from build123d import *

# Parameters (mm, degrees)
SKETCH_1_R          = 42.5
SKETCH_1_R_2        = 3
EXTRUDE_1_DEPTH     = 6
SKETCH_1_3_R        = 42.5
SKETCH_1_3_R_2      = 37.5
EXTRUDE_2_DEPTH     = 62
EXTRUDE_START       = 37
SKETCH_1_5_R        = 37.5
SKETCH_1_5_R_2      = 20
EXTRUDE_3_DEPTH     = 5
CHAMFER_1_SIZE      = 2
EXTRUDE_4_DEPTH     = 37
CUT_EXTRUDE_2_DEPTH = 25
CUT_EXTRUDE_3_REACH = 78.25


with BuildPart() as part:
    # 草图1 → 凸台-拉伸1 (new body)
    with BuildSketch(Plane(origin=(0, 0, 0), x_dir=(1, 0, 0), z_dir=(0, 1, 0))):
        with BuildLine():
            Line((-36, 45), (36, 45))
            ThreePointArc((36, 45), (42.363961031, 42.363961031), (45, 36))
            Line((45, 36), (45, -36))
            ThreePointArc((45, -36), (42.363961031, -42.363961031), (36, -45))
            Line((36, -45), (-36, -45))
            ThreePointArc((-36, -45), (-42.363961031, -42.363961031), (-45, -36))
            Line((-45, -36), (-45, 36))
            ThreePointArc((-45, 36), (-42.363961031, 42.363961031), (-36, 45))
        make_face()
        with Locations(Location((0, 0, 0), (0, 0, 270))):
            Circle(SKETCH_1_R, mode=Mode.SUBTRACT)
        with Locations(Location((-36, 36, 0), (0, 0, 270))):
            Circle(SKETCH_1_R_2, mode=Mode.SUBTRACT)
        with Locations(Location((36, 36, 0), (0, 0, 270))):
            Circle(SKETCH_1_R_2, mode=Mode.SUBTRACT)
        with Locations(Location((36, -36, 0), (0, 0, 270))):
            Circle(SKETCH_1_R_2, mode=Mode.SUBTRACT)
        with Locations(Location((-36, -36, 0), (0, 0, 270))):
            Circle(SKETCH_1_R_2, mode=Mode.SUBTRACT)
    extrude(amount=EXTRUDE_1_DEPTH)

    # 草图1<3> → 凸台-拉伸2 (add)
    with BuildSketch(Plane(origin=(0, 0, 0), x_dir=(1, 0, 0), z_dir=(0, 1, 0))):
        with Locations(Location((0, 0, 0), (0, 0, 270))):
            Circle(SKETCH_1_3_R)
        with Locations(Location((0, 0, 0), (0, 0, 270))):
            Circle(SKETCH_1_3_R_2, mode=Mode.SUBTRACT)
    extrude(amount=EXTRUDE_2_DEPTH)

    # 草图1<5> → 凸台-拉伸3 (add)
    with BuildSketch(Plane(origin=(0, 0, 0), x_dir=(1, 0, 0), z_dir=(0, 1, 0)).offset(EXTRUDE_START)):
        with Locations(Location((0, 0, 0), (0, 0, 270))):
            Circle(SKETCH_1_5_R)
        with Locations(Location((0, 0, 0), (0, 0, 270))):
            Circle(SKETCH_1_5_R_2, mode=Mode.SUBTRACT)
    extrude(amount=EXTRUDE_3_DEPTH)

    # 倒角1
    chamfer_1_edges = [part.edges().sort_by_distance(p)[0] for p in [
        (0, 42, -20),
    ]]
    chamfer(chamfer_1_edges, length=CHAMFER_1_SIZE)

    # 草图1<6> → 凸台-拉伸4 (add)
    with BuildSketch(Plane(origin=(0, 0, 0), x_dir=(1, 0, 0), z_dir=(0, 1, 0))):
        with BuildLine():
            Line((27.950849719, -25), (-27.950849719, -25))
            ThreePointArc((-27.950849719, -25), (0, -37.5), (27.950849719, -25))
        make_face()
    extrude(amount=EXTRUDE_4_DEPTH)

    # 草图2 → 切除-拉伸2 (cut)
    with BuildSketch(Plane(origin=(0, 6, 0), x_dir=(1, 0, 0), z_dir=(0, 1, 0))):
        with BuildLine():
            Line((-27.882352941, -27.978999168), (-30, -30.103986447))
            ThreePointArc((-30, -30.103986447), (0, -42.5), (30, -30.103986447))
            Line((30, -30.103986447), (27.882352941, -27.978999168))
            ThreePointArc((27.882352941, -27.978999168), (0, -39.5), (-27.882352941, -27.978999168))
        make_face()
    extrude(amount=CUT_EXTRUDE_2_DEPTH, mode=Mode.SUBTRACT)

    # 草图3 → 切除-旋转1 (revolve, cut)
    with BuildSketch(Plane(origin=(0, 18.5, 0), x_dir=(1, 0, 0), z_dir=(0, 1, 0))):
        Polygon((11.657691454, -25), (17.095538176, -22.46429043), (18.961631098, -26.466139615), (15.789553843, -27.945303531), (20.195943791, -37.394837269), (17.930174324, -38.451382923), align=None)
    revolve(axis=Axis((17.930174324, 18.5, 38.451382923), (-0.42261826174070033, 0, -0.9063077870366495)), mode=Mode.SUBTRACT)

    # 草图3<4> → 切除-旋转2 (revolve, cut)
    with BuildSketch(Plane(origin=(0, 18.5, 0), x_dir=(1, 0, 0), z_dir=(0, 1, 0)), mode=Mode.PRIVATE) as cut_revolve_2_sk:
        Polygon((-20.195943791, -37.394837269), (-17.930174324, -38.451382923), (-11.657691454, -25), (-17.095538176, -22.46429043), (-18.961631098, -26.466139615), (-15.789553843, -27.945303531), align=None)
    revolve(cut_revolve_2_sk.sketch.rotate(Axis((-17.930174324, 18.5, 38.451382923), (0.42261826174069994, 0, -0.9063077870366497)), 180), axis=Axis((-17.930174324, 18.5, 38.451382923), (0.42261826174069994, 0, -0.9063077870366497)), mode=Mode.SUBTRACT)

    # 草图5 → 切除-拉伸3 (cut, up to next)
    with BuildSketch(Plane(origin=(0, 42, 0), x_dir=(1, 0, 0), z_dir=(0, 1, 0)), mode=Mode.PRIVATE) as cut_extrude_3_sk1:
        with BuildLine():
            Line((-6, 30), (-2.872281323, 30))
            ThreePointArc((-2.872281323, 30), (0, 31.5), (2.872281323, 30))
            Line((2.872281323, 30), (6, 30))
            ThreePointArc((6, 30), (8, 28), (6, 26))
            Line((6, 26), (2.872281323, 26))
            ThreePointArc((2.872281323, 26), (0, 24.5), (-2.872281323, 26))
            Line((-2.872281323, 26), (-6, 26))
            ThreePointArc((-6, 26), (-8, 28), (-6, 30))
        make_face()
    cut_extrude_3_tool1 = extrude(cut_extrude_3_sk1.sketch, amount=-CUT_EXTRUDE_3_REACH, mode=Mode.PRIVATE) & part.part
    # 草图5 → 切除-拉伸3 (cut, up to next)
    with BuildSketch(Plane(origin=(0, 42, 0), x_dir=(1, 0, 0), z_dir=(0, 1, 0)), mode=Mode.PRIVATE) as cut_extrude_3_sk2:
        with BuildLine():
            Line((26, 6), (26, 2.872281323))
            ThreePointArc((26, 2.872281323), (24.5, 0), (26, -2.872281323))
            Line((26, -2.872281323), (26, -6))
            ThreePointArc((26, -6), (28, -8), (30, -6))
            Line((30, -6), (30, -2.872281323))
            ThreePointArc((30, -2.872281323), (31.5, 0), (30, 2.872281323))
            Line((30, 2.872281323), (30, 6))
            ThreePointArc((30, 6), (28, 8), (26, 6))
        make_face()
    cut_extrude_3_tool2 = extrude(cut_extrude_3_sk2.sketch, amount=-CUT_EXTRUDE_3_REACH, mode=Mode.PRIVATE) & part.part
    # 草图5 → 切除-拉伸3 (cut, up to next)
    with BuildSketch(Plane(origin=(0, 42, 0), x_dir=(1, 0, 0), z_dir=(0, 1, 0)), mode=Mode.PRIVATE) as cut_extrude_3_sk3:
        with BuildLine():
            Line((-26, -6), (-26, -2.872281323))
            ThreePointArc((-26, -2.872281323), (-24.5, 0), (-26, 2.872281323))
            Line((-26, 2.872281323), (-26, 6))
            ThreePointArc((-26, 6), (-28, 8), (-30, 6))
            Line((-30, 6), (-30, 2.872281323))
            ThreePointArc((-30, 2.872281323), (-31.5, 0), (-30, -2.872281323))
            Line((-30, -2.872281323), (-30, -6))
            ThreePointArc((-30, -6), (-28, -8), (-26, -6))
        make_face()
    cut_extrude_3_tool3 = extrude(cut_extrude_3_sk3.sketch, amount=-CUT_EXTRUDE_3_REACH, mode=Mode.PRIVATE) & part.part
    add(cut_extrude_3_tool1.solids().sort_by_distance((0, 42, -28))[0], mode=Mode.SUBTRACT)
    add(cut_extrude_3_tool2.solids().sort_by_distance((28, 42, 0))[0], mode=Mode.SUBTRACT)
    add(cut_extrude_3_tool3.solids().sort_by_distance((-28, 42, 0))[0], mode=Mode.SUBTRACT)


solid = part.part
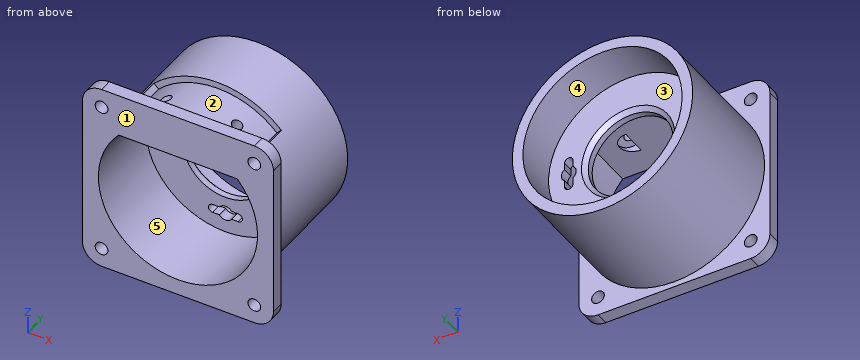
Input: part model. Units: mm. Frame: model coordinates. Face numbers are marked on the shaded views. A direction names the side the tool comes from. Give positions to 0.01 mm unless a question says otherwise; leave off trailing zeros. Order: outer loops, then holes, each group sorted by start corner. A loop starts at its lowest first (then second) coordinate and runs counter-clockwise, first axis right, second up. Notation, with made-up numbers: (85, -16) - (105, -16) arc R29 ccw to (105, 14) - close; hole circle Ø8 at (58, -22). An arc over 180 degrees is marked (long way). Answer as a JSON object with one key per item and string values. Group by question number.
Q1. Cut plane D-D, the plane y = 14. Output: boundary loops of the cut face in (x, z).
Q2. Cut plane A-A, the plane x = 0. Output: boundary loops of the cut face in (y, z).
Q3. Cut plane C-C, the plane y = 32.5. Output: boundary loops of the cut face in (x, z).
Q4. Line query: probe 1 along X at (y, z) = (1, 36); probe 2 along X at (y, z) = (22, 0); probe 3 along Y at (x, z) = (12.5, 40). Output: solid intervals per line, ascending.
Q5. First-contact query: pin 1 Ø3.5 at (y, z) = (39, -4.5) entering from -X; pin 2 Ø0.9 at (x, y) = (3.5, 40.5) entering from -Z; pin 3 Ø0.9 at (y, z) = (40, -5) entering from +X; pin 4 Ø5 at (x, z) = (-36, -36) entering from +Y. Flat tips, straight axial feed; report the tip coordinate or a pass-through.
Q6. Mould query, pull axis Z, two halves, no side actions, for the marked faces 1, 2 and 3. Classes: pulls with the +Z half, pulls with the -Z half, needs draft (parallel to the pull), parting line crosses it, or undercut.
Q7. Set-up query: the marked faces 4 and 5. Return all of +Z, -Z, +X, -X, +Y, -Y with unobstructed straight access to the full face (end or side cutting, diameter ignored); none if empty.
Q8. Cut plane B-B, the plane z = -28. Output: boundary loops of the cut face in (x, y), then the cut area to 3 significant figures.
Results:
{
 "1": {"outline": "(-30, 30.1) arc R42.5 ccw (long way) to (30, 30.1) - (27.88, 27.98) arc R39.5 ccw to (-27.88, 27.98) - close; hole (-27.95, 25) arc R37.5 ccw (long way) to (27.95, 25) - (16.04, 25) - (17.12, 27.32) - (9.93, 30.68) - (8.06, 26.68) - (11.66, 25) - (-11.66, 25) - (-8.06, 26.68) - (-9.93, 30.68) - (-17.12, 27.32) - (-16.04, 25) - close"},
 "2": {"outline": "(0, -45) - (6, -45) - (6, -42.5) - (62, -42.5) - (62, -37.5) - (42, -37.5) - (42, -31.5) - (37, -31.5) - (37, -37.5) - (0, -37.5) - close; (0, 25) - (37, 25) - (37, 20) - (40, 20) - (42, 22) - (42, 37.5) - (62, 37.5) - (62, 42.5) - (31, 42.5) - (31, 39.5) - (6, 39.5) - (6, 45) - (0, 45) - close; (37, -24.5) - (42, -24.5) - (42, -22) - (40, -20) - (37, -20) - close"},
 "3": {"outline": "circle Ø85 at (0, 0); hole (-27.95, 25) arc R37.5 ccw (long way) to (27.95, 25) - close"},
 "4": {"probe 1": "-45 to -39, -33 to 33, 39 to 45", "probe 2": "-42.5 to -37.5, 37.5 to 42.5", "probe 3": "0 to 6, 31 to 62"},
 "5": {"pin 1": "x = -42.41", "pin 2": "z = -42.39", "pin 3": "x = 42.26", "pin 4": "through"},
 "6": {"face 1": "needs draft", "face 2": "pulls with the +Z half", "face 3": "undercut"},
 "7": {"face 4": "+Y", "face 5": "-Y"},
 "8": {"outline": "(-45, 0) - (-24.94, 0) - (-24.94, 37) - (-8, 37) - (-8, 42) - (-24.94, 42) - (-24.94, 62) - (-31.97, 62) - (-31.97, 6) - (-45, 6) - close; (8, 37) - (24.94, 37) - (24.94, 0) - (45, 0) - (45, 6) - (31.97, 6) - (31.97, 62) - (24.94, 62) - (24.94, 42) - (8, 42) - close", "area": "1,200 mm^2"}
}
